Source: CAD feature listing. Evaluate the final solid. Frame: model axes, mm. Face numbers are marked on the shaded views. A direction names the side the tool comes from. Coordinates: 2 decimals unless noted, no trailing zeros. Write each loop counter-clockwise with the first axis right and the second up, starting at its lowest first coordinate (ties: lowest second). Pieces come first, ordered by that corner, then holes. Notation, with made-up numbers: M 69.5,3.25 L 103.5,3.25 A11 cw 103.5,22.25 Z; hole C -11,-31.5 d6. An arc over 180 degrees is marked long. Write item = value, one per line. Start each with the question number.
1. Section query D-D (z = 21.5). Output: boundary loops of the cut face in (x, y).
2. Access query for the marked faces 5, 6, 7 and 8. Directions: +Z, -Z, +X, -X, +Y, -Y. A direction counts if a zero-diameter tool reaches every point of the face in a straight line with its end or side. Return the directions, or none.
3. Section query B-B (y = -48). Output: boundary loops of the cut face in (x, z), then the cut area to 4 significant figures.
4. Line query: line 1 along X through (y, z) = (-32, 5); line 2 along Y through (x, z) = (-31, 35); line 3 along X through (y, z) = (28, 23.5). Output: solid intervals per line, ascending.
5. Pin query (flat end, axial travel): pin 1 Ø4.5 at (x, z) = (19, 3) entering from -Y; pin 2 Ø1 at (y, z) = (26.5, 24.5) entering from -X; pin 3 Ø5 at (x, z) = (20.5, 33) entering from +Y. Return the tip coordinate at first contact, or that it passes through.
6. Pull-direction query (Y, two-part tool) for the marked faces 1, 2, 3 and 4; classes: pulls with the +Y half, pulls with the -Y half, needs draft (parallel to the pull), parting line crosses it, or undercut.
7. Section query C-C (z = 4.5). Output: boundary loops of the cut face in (x, y), then the cut area to 3 significant figures.
8. Section query A-A (x = -2). Output: boundary loops of the cut face in (y, z), then the cut area to 3 significant figures.
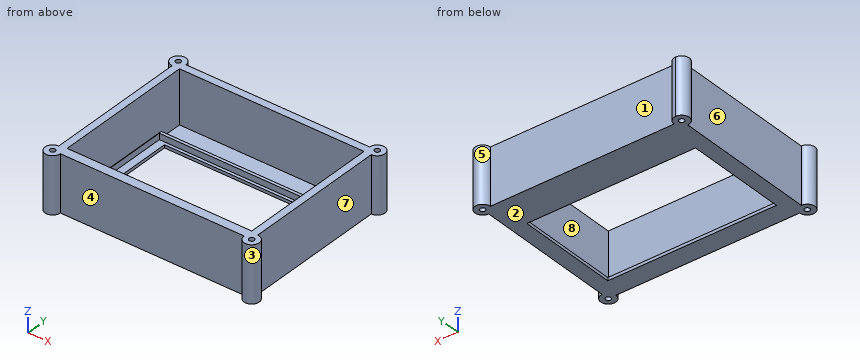
```python
from build123d import *

# Parameters (mm, degrees)
F0_W     = 121
F0_H     = 76
F0_W_2   = 111
F0_H_2   = 67
F1_DEPTH = 2
F2_DEPTH = 6
F0_W_3   = 121.5
F0_H_3   = 15
F3_DEPTH = 2
F0_R     = 1.75
F4_DEPTH = 37


with BuildPart() as f1:
    # F0 (on Top) → F1 (new body)
    with BuildSketch(Plane.XY):
        with Locations((-8.830484, -22.025124)):
            Rectangle(F0_W, F0_H)
        with Locations((-8.830484, -19.525124)):
            Rectangle(F0_W_2, F0_H_2, mode=Mode.SUBTRACT)
    extrude(amount=F1_DEPTH)

    # F0 (on Top) → F2 (join)
    with BuildSketch(Plane.XY):
        Polygon((-69.580484, -60.025124), (-69.330484, -60.025124), (-69.330484, 15.974876), (51.669516, 15.974876), (51.669516, -60.025124), (51.919516, -60.025124), (51.919516, 17.974876), (-69.580484, 17.974876), align=None)
    extrude(amount=F2_DEPTH)

    # F0 (on Top) → F3 (join)
    with BuildSketch(Plane.XY):
        with Locations((-8.830484, 25.474876)):
            Rectangle(F0_W_3, F0_H_3)
    extrude(amount=F3_DEPTH)

    # F0 (on Top) → F4 (join)
    with BuildSketch(Plane.XY):
        with BuildLine():
            Line((-74.330484, 32.974876), (-69.580484, 32.974876))
            Line((-69.580484, 32.974876), (51.919516, 32.974876))
            Line((51.919516, 32.974876), (56.669516, 32.974876))
            ThreePointArc((56.669516, 32.974876), (60.20505, 41.51041), (51.669516, 37.974876))
            Line((51.669516, 37.974876), (-69.330484, 37.974876))
            ThreePointArc((-69.330484, 37.974876), (-70.796105, 41.511565), (-74.333752, 42.974875))
            ThreePointArc((-74.333752, 42.974875), (-79.330483, 37.973242), (-74.330484, 32.974876))
        make_face()
        with Locations((-74.330484, 37.974876)):
            Circle(F0_R, mode=Mode.SUBTRACT)
        with Locations((56.669516, 37.974876)):
            Circle(F0_R, mode=Mode.SUBTRACT)
        with BuildLine():
            Line((51.669516, -60.025124), (-69.330484, -60.025124))
            Line((-69.330484, -60.025124), (-69.580484, -60.025124))
            Line((-69.580484, -60.025124), (-69.580484, 17.974876))
            Line((-69.580484, 17.974876), (-69.580484, 32.974876))
            Line((-69.580484, 32.974876), (-74.330484, 32.974876))
            Line((-74.330484, 32.974876), (-74.330484, -61.025124))
            ThreePointArc((-74.330484, -61.025124), (-77.866018, -69.560658), (-69.330484, -66.025124))
            Line((-69.330484, -66.025124), (51.669516, -66.025124))
            ThreePointArc((51.669516, -66.025124), (60.20505, -69.560658), (56.669516, -61.025124))
            Line((56.669516, -61.025124), (56.669516, 32.974876))
            Line((56.669516, 32.974876), (51.919516, 32.974876))
            Line((51.919516, 32.974876), (51.919516, 17.974876))
            Line((51.919516, 17.974876), (51.919516, -60.025124))
            Line((51.919516, -60.025124), (51.669516, -60.025124))
        make_face()
        with Locations((-74.330484, -66.025124)):
            Circle(F0_R, mode=Mode.SUBTRACT)
        with Locations((56.669516, -66.025124)):
            Circle(F0_R, mode=Mode.SUBTRACT)
    extrude(amount=F4_DEPTH)


solid = f1.part
```
Results are:
q1.outline = M -74.33,-61.03 A5 ccw long -69.33,-66.03 L 51.67,-66.03 A5 ccw long 56.67,-61.03 L 56.67,32.97 A5 ccw long 51.67,37.97 L -69.33,37.97 A5 ccw long -74.33,32.97 Z; hole C -74.33,-66.03 d3.5; hole C -74.33,37.97 d3.5; hole M -69.58,-60.03 L 51.92,-60.03 L 51.92,32.97 L -69.58,32.97 Z; hole C 56.67,-66.03 d3.5; hole C 56.67,37.97 d3.5
q2.face_5 = +Z, -Z
q2.face_6 = +Z, -Z, -X
q2.face_7 = +Z, -Z, +X
q2.face_8 = +Z
q3.outline = M -74.33,0 L -64.33,0 L -64.33,2 L -69.33,2 L -69.33,6 L -69.58,6 L -69.58,37 L -74.33,37 Z; M 46.67,0 L 56.67,0 L 56.67,37 L 51.92,37 L 51.92,6 L 51.67,6 L 51.67,2 L 46.67,2 Z
q3.area = 374.5 mm^2
q4.line_1 = -74.33 to -69.33, 51.67 to 56.67
q4.line_2 = -66.03 to -60.03, 32.97 to 37.97
q4.line_3 = -74.33 to -69.58, 51.92 to 56.67
q5.pin_1 = -66.03
q5.pin_2 = -74.33
q5.pin_3 = 37.97
q6.face_1 = pulls with the +Y half
q6.face_2 = needs draft
q6.face_3 = undercut
q6.face_4 = pulls with the -Y half
q7.outline = M -74.33,-61.03 A5 ccw long -69.33,-66.03 L 51.67,-66.03 A5 ccw long 56.67,-61.03 L 56.67,32.97 A5 ccw long 51.67,37.97 L -69.33,37.97 A5 ccw long -74.33,32.97 Z; hole C -74.33,-66.03 d3.5; hole C -74.33,37.97 d3.5; hole M -69.58,17.97 L 51.92,17.97 L 51.92,32.97 L -69.58,32.97 Z; hole M -69.33,-60.03 L 51.67,-60.03 L 51.67,15.97 L -69.33,15.97 Z; hole C 56.67,-66.03 d3.5; hole C 56.67,37.97 d3.5
q7.area = 2,800 mm^2
q8.outline = M -66.03,0 L -53.03,0 L -53.03,2 L -60.03,2 L -60.03,37 L -66.03,37 Z; M 13.97,0 L 37.97,0 L 37.97,37 L 32.97,37 L 32.97,2 L 17.97,2 L 17.97,6 L 15.97,6 L 15.97,2 L 13.97,2 Z
q8.area = 467 mm^2
